Geometry check sheet. Reference: drawing and pictorial views, mm from the part's lowest x, y, z. A direction names the side the tool comes from. Round coordinates to 2 decimals unless told otherwise and drop trailing zeros. Write each loop counter-clockwise with the first axis right and the second up, starting at its lowest first coordinate (ties: lowest second). Pieces come first, ordered by that corner, then holes.
Item 1: Section check D-D, the plane x = 11. Record the cut outline in (y, z) (3 decimals), plus the area to 3 significant figures.
Item 2: Release check for a two-part mould opening along Z. For the marked faces 1, 2 and 3 record: pulls with the +Z half, pulls with the -Z half, needs draft (parallel to the pull), parting line crosses it, or undercut.
Item 3: Set-up check for the marked faces 4, 5 and 6: record each of +Z, -Z, +X, -X, +Y, -Y from which the full face is reachable in a straight line by a thin tool's end or side.
Item 4: Depth check by flat-ended pin: pin 1 (8.5 mm diameter, centred on x = 40, z = 5.5, fed in from -Y); pin 2 (1 mm diameter, centred on x = 31.5, z = 15, fed in from +Y); pin 3 (10 mm diameter, centred on x = 24.5, z = 8.5, fed in from -Y); pin 4 (8 mm diameter, centred on y = 4.5, z = 9.5, fed in from -X). Enter the tip coordinate at first touch or a pass-through.
Item 5: Section check A-A, the plane y = 12. Record the cut outline in (x, z), plus the area to 3 significant figures.
Item 6: Section check C-C, the plane z = 18. Record the cut outline in (x, y), plus the area to 3 significant figures.
Item 7: Section check B-B, the plane y = 4.25. Record the cut outline in (x, z) (3 decimals).
Item 8: Material ranges on line 1 along X through (y, z) = (1.5, 13.75); line 2 along X through (y, z) = (14, 13.25); line 3 along Y through (x, z) = (42.5, 5), recorded low to high.
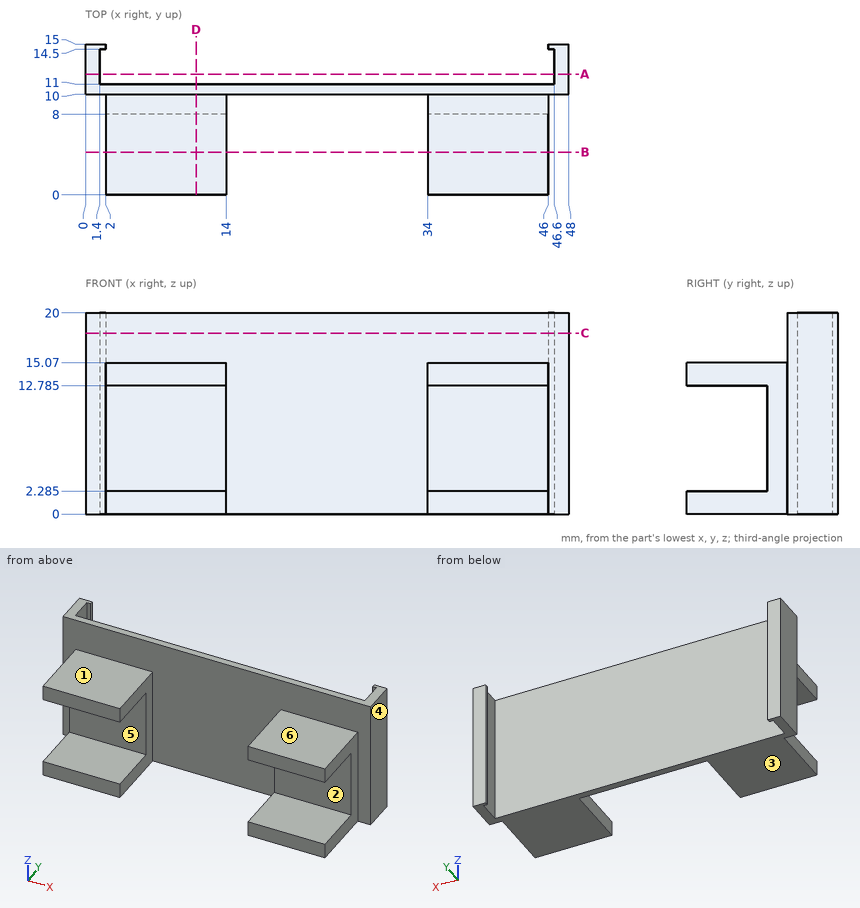
Values found:
1. outline: (0, 0) - (11, 0) - (11, 20) - (10, 20) - (10, 15.07) - (0, 15.07) - (0, 12.785) - (8, 12.785) - (8, 2.285) - (0, 2.285) - close
1. area: 86.7 mm2
2. face 1: pulls with the +Z half
2. face 2: undercut
2. face 3: pulls with the -Z half
3. face 4: +Z, -Z, +X, +Y, -Y
3. face 5: +X, -X, -Y
3. face 6: +Z, +X, -X, -Y
4. pin 1: stops at y = 0
4. pin 2: stops at y = 11
4. pin 3: stops at y = 10
4. pin 4: stops at x = 2
5. outline: (0, 0) - (1.4, 0) - (1.4, 20) - (0, 20) - close; (46.6, 0) - (48, 0) - (48, 20) - (46.6, 20) - close
5. area: 56.0 mm2
6. outline: (0, 10) - (48, 10) - (48, 15) - (46, 15) - (46, 14.5) - (46.6, 14.5) - (46.6, 11) - (1.4, 11) - (1.4, 14.5) - (2, 14.5) - (2, 15) - (0, 15) - close
6. area: 59.8 mm2
7. outline: (2, 0) - (14, 0) - (14, 2.285) - (2, 2.285) - close; (2, 12.785) - (14, 12.785) - (14, 15.07) - (2, 15.07) - close; (34, 0) - (46, 0) - (46, 2.285) - (34, 2.285) - close; (34, 12.785) - (46, 12.785) - (46, 15.07) - (34, 15.07) - close
8. line 1: x = 2 to 14, 34 to 46
8. line 2: x = 0 to 1.4, 46.6 to 48
8. line 3: y = 8 to 11
